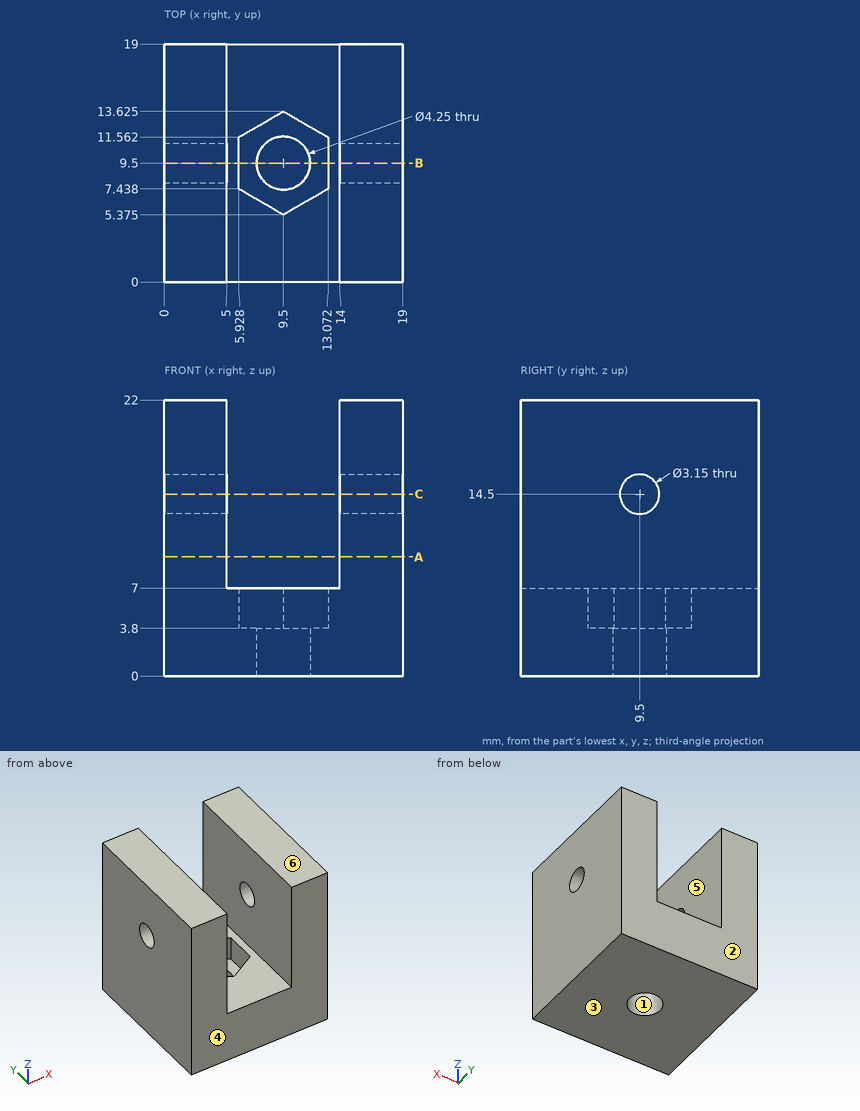
Study the drawing (mm; zero at the part's minimum x, y, z) and answer. A direction names the side the tool comes from. Give positions to 0.01 mm unless a question says otherwise; leave off trailing zeros. Loops run counter-clockwise (first coordinate to the right, second up) from the corner with the lowest first, then second, coordinate; pieces in that order, holes last. Notation, with made-up numbers: (66.5, 40) - (84.5, 40) arc R22 cw to (84.5, 65) - close; hole circle Ø7 at (38.25, 20). An arc over 180 degrees is marked (long way). Return JSON: item names as keys, results as strings. Group by question number.
1. Given pin 1 Ø2.5 at (x, y) = (8, 13.5) entering from +Z; pin 2 Ø1 at (x, z) = (12.5, 16.5) entering from +Y; pin 3 Ø5.5 at (x, y) = (9.5, 9.5) entering from +Z, each flat-ended and moving along its own axis, determine where each tip first touches the part or whether it passes through.
2. Determine the mould class of the marked faces 1, 2, 3 and 4 for opening direction Y: pulls with the +Y half, pulls with the -Y half, needs draft (parallel to the pull), parting line crosses it, or undercut.
3. Straight lines are drawn through the part: line 1 (X direction, y = 8, z = 19.25); line 2 (X direction, y = 9.5, z = 1.35) (1 decimal); line 3 (Y direction, x = 2.15, z = 14.5) (1 decimal). For each, find the intervals that lie inside material, in ascending order. Write a range as [from, to].
4. Find section A-A (z = 9.5). Write down the section's boundary in (x, y), then the cut area to 3 significant figures.
5. Find section C-C (z = 14.5). Write down the section's boundary in (x, y) (1 decimal).
6. Which of the six approach directions +Z, -Z, +X, -X, +Y, -Y give full straight-line access (tool end or side, diameter ignored) to the marked faces 5 and 6?
7. Find section B-B (y = 9.5). Write down the section's boundary in (x, z) (1 decimal).
Verdict:
{
 "1": {"pin 1": "stops at z = 7", "pin 2": "passes through", "pin 3": "stops at z = 3.8"},
 "2": {"face 1": "undercut", "face 2": "pulls with the +Y half", "face 3": "needs draft", "face 4": "pulls with the -Y half"},
 "3": {"line 1": "x = [0, 5], [14, 19]", "line 2": "x = [0, 7.4], [11.6, 19]", "line 3": "y = [0, 7.9], [11.1, 19]"},
 "4": {"outline": "(0, 0) - (5, 0) - (5, 19) - (0, 19) - close; (14, 0) - (19, 0) - (19, 19) - (14, 19) - close", "area": "190 mm^2"},
 "5": {"outline": "(0, 0) - (5, 0) - (5, 7.9) - (0, 7.9) - close; (0, 11.1) - (5, 11.1) - (5, 19) - (0, 19) - close; (14, 0) - (19, 0) - (19, 7.9) - (14, 7.9) - close; (14, 11.1) - (19, 11.1) - (19, 19) - (14, 19) - close"},
 "6": {"face 5": "+Z, +Y, -Y", "face 6": "+Z, +X, -X, +Y, -Y"},
 "7": {"outline": "(0, 0) - (7.4, 0) - (7.4, 3.8) - (5.9, 3.8) - (5.9, 7) - (5, 7) - (5, 12.9) - (0, 12.9) - close; (0, 16.1) - (5, 16.1) - (5, 22) - (0, 22) - close; (11.6, 0) - (19, 0) - (19, 12.9) - (14, 12.9) - (14, 7) - (13.1, 7) - (13.1, 3.8) - (11.6, 3.8) - close; (14, 16.1) - (19, 16.1) - (19, 22) - (14, 22) - close"}
}
